Solid Edge part; units mm, degrees
sketch "Sketch1" plane through (0, 0, 0) normal (0, 0, 1) x (1, 0, 0)
  line L0 (-50, -50) -> (50, -50)
  line L1 (50, -50) -> (50, 50)
  line L2 (50, 50) -> (-50, 50)
  line L3 (-50, 50) -> (-50, -50)
extrude "Protrusion1" add sketch "Sketch1" along normal blind 3
sketch "Sketch2" plane through (0, 0, 3) normal (0, 0, 1) x (1, 0, 0)
  circle A0 centre (31.5, 45) radius 1.7293
  circle A1 centre (31.5, -4) radius 1.7293
  circle A2 centre (-26.5, -4) radius 1.7293
  line L0 (-40, 1) -> (31.5, 1)
  line L1 (31.5, 1) -> (31.5, 40)
  line L2 (31.5, 40) -> (-40, 40)
  line L3 (-40, 40) -> (-40, 1)
  circle A3 centre (-26.5, 45) radius 1.7293
  line L4 (-40, -45) -> (31.5, -45)
  line L5 (31.5, -45) -> (31.5, -9)
  line L6 (31.5, -9) -> (-40, -9)
  line L7 (-40, -9) -> (-40, -45)
  dimension "D1" = 26.5
extrude "ExtrudedCutout_1" cut sketch "Sketch2" against normal blind 3
sketch "Sketch3" plane through (0, 0, 3) normal (0, 0, 1) x (0, 1, 0)
  line L0 (50, 50) -> (50, 40)
  line L1 (47, 40) -> (50, 40)
  line L2 (47, 50) -> (47, 40)
  line L3 (50, 50) -> (47, 50)
  line L4 (50, -40) -> (47, -40)
  line L5 (47, -40) -> (47, -50)
  line L6 (47, -50) -> (50, -50)
  line L7 (50, -50) -> (50, -40)
  line L8 (-50, -50) -> (-47, -50)
  line L9 (-47, -50) -> (-47, -40)
  line L10 (-47, -40) -> (-50, -40)
  line L11 (-50, -40) -> (-50, -50)
  line L12 (-50, 40) -> (-47, 40)
  line L13 (-47, 40) -> (-47, 50)
  line L14 (-47, 50) -> (-50, 50)
  line L15 (-50, 50) -> (-50, 40)
extrude "ExtrudedProtrusion_2" add sketch "Sketch3" along normal blind 5
fillet "Round_1" radius 3 8 edges at (-40, 48.5, 8) (-50, 48.5, 8) (50, 48.5, 8) (40, 48.5, 8) (50, -48.5, 8) (40, -48.5, 8) (-40, -48.5, 8) (-50, -48.5, 8)
fillet "Round_2" radius 1 12 edges at (-40, 20.5, 3) (-4.25, 40, 3) (31.5, 20.5, 3) (-4.25, 1, 3) (-40, -27, 3) (-4.25, -9, 3) (50, 0, 3) (0, -50, 3) (-4.25, -45, 3) (31.5, -27, 3) (0, 50, 3) (-50, 0, 3)
Build history of the part. All positions in model axes, mm. Round coordinates to 2 decimals unless told otherwise and drop trailing zeros. Order: outer loops, then holes, each group sorted by start corner. A loop starts at its lowest first (then second) coordinate and runs counter-clockwise, first axis right, second up. Notation, with made-up numbers: (-18.75, 47) -> (-7.75, 47) arc R10 ccw to (-7.75, 58) -> close; hole circle Ø6 at (71, 30). An arc over 180 degrees is marked (long way). Answer in a Markdown table with one row per item.
1) Band-saw the part on D-D on y = 45. Give the cut face in (x, z).
Values:
| item | result |
|---|---|
| outline | (-50, 0) -> (-28.23, 0) -> (-28.23, 3) -> (-49, 3) arc R1 ccw to (-50, 2) -> close; (-24.77, 0) -> (29.77, 0) -> (29.77, 3) -> (-24.77, 3) -> close; (33.23, 0) -> (50, 0) -> (50, 2) arc R1 ccw to (49, 3) -> (33.23, 3) -> close |
2) Pin check, flat tip, straight feed: P1, Ø4, axis at x = -26.5, y = 45, coming from the +Z side. Stop position of the tip, or through.
Values:
| item | result |
|---|---|
| P1 | z = 3 |
3) Band-saw the part on A-A on x = -26.5. Give the cut face in (y, z).
Values:
| item | result |
|---|---|
| outline | (-50, 0) -> (-45, 0) -> (-45, 2) arc R1 ccw to (-46, 3) -> (-49, 3) arc R1 ccw to (-50, 2) -> close; (-9, 0) -> (-5.73, 0) -> (-5.73, 3) -> (-8, 3) arc R1 ccw to (-9, 2) -> close; (-2.27, 0) -> (1, 0) -> (1, 2) arc R1 ccw to (0, 3) -> (-2.27, 3) -> close; (40, 0) -> (43.27, 0) -> (43.27, 3) -> (41, 3) arc R1 ccw to (40, 2) -> close; (46.73, 0) -> (50, 0) -> (50, 2) arc R1 ccw to (49, 3) -> (46.73, 3) -> close |
4) Mould opens along X. For faces 1 (the cylindrical face through (-40.9, 48.52, 7.14)), 2 (the flat face through (45, -47, 6)), 3 (the cylindrical face through (-49.1, 48.48, 7.14)) say: released by +X, released by -X, zero draft, split by the parting line, or undercut.
Values:
| item | result |
|---|---|
| face 1 | undercut |
| face 2 | zero draft |
| face 3 | released by -X |
5) Band-saw the part on C-C on x = 19. Give the cut face in (y, z), and give its area (3 significant figures).
Values:
| item | result |
|---|---|
| outline | (-50, 0) -> (-45, 0) -> (-45, 2) arc R1 ccw to (-46, 3) -> (-49, 3) arc R1 ccw to (-50, 2) -> close; (-9, 0) -> (1, 0) -> (1, 2) arc R1 ccw to (0, 3) -> (-8, 3) arc R1 ccw to (-9, 2) -> close; (40, 0) -> (50, 0) -> (50, 2) arc R1 ccw to (49, 3) -> (41, 3) arc R1 ccw to (40, 2) -> close |
| area | 73.7 mm2 |
6) Wall check: L1, parallel to Y at x = -17, z = 2; L2, parallel to X at y = 7.5, z = 1.75; L3, parallel to Y at x = -26.5, z = 1.6. Give the ranges that are in metal, low to high.
Values:
| item | result |
|---|---|
| L1 | -50 to -45, -9 to 1, 40 to 50 |
| L2 | -50 to -40, 31.5 to 50 |
| L3 | -50 to -45, -9 to -5.73, -2.27 to 1, 40 to 43.27, 46.73 to 50 |
7) Band-saw the part on B-B on y = -41. Give the cut face in (x, z).
Values:
| item | result |
|---|---|
| outline | (-50, 0) -> (-40, 0) -> (-40, 2) arc R1 ccw to (-41, 3) -> (-49, 3) arc R1 ccw to (-50, 2) -> close; (31.5, 0) -> (50, 0) -> (50, 2) arc R1 ccw to (49, 3) -> (32.5, 3) arc R1 ccw to (31.5, 2) -> close |
